from build123d import *

# Parameters (mm, degrees)
SKETCH1_R           = 22.25
BOSS_EXTRUDE1_DEPTH = 67.5
SKETCH2_R           = 8.75
BOSS_EXTRUDE2_DEPTH = 4.7
SKETCH3_R           = 2.5
BOSS_EXTRUDE3_DEPTH = 14.5
SKETCH4_R           = 2
CUT_EXTRUDE1_DEPTH  = 14.5
FILLET1_R           = 2
FILLET2_R           = 1


with BuildPart() as part:
    # Sketch1 → Boss-Extrude1 (new body)
    with BuildSketch(Plane(origin=(0, 0, 0), x_dir=(1, 0, 0), z_dir=(0, 1, 0))):
        with Locations(Location((0, 0, 0), (0, 0, 270))):
            Circle(SKETCH1_R)
    extrude(amount=BOSS_EXTRUDE1_DEPTH)

    # Sketch2 → Boss-Extrude2 (add)
    with BuildSketch(Plane(origin=(0, 67.5, 0), x_dir=(1, 0, 0), z_dir=(0, 1, 0))):
        with Locations(Location((0, 0, 0), (0, 0, 270))):
            Circle(SKETCH2_R)
    extrude(amount=BOSS_EXTRUDE2_DEPTH)

    # Sketch3 → Boss-Extrude3 (add)
    with BuildSketch(Plane(origin=(0, 72.2, 0), x_dir=(1, 0, 0), z_dir=(0, 1, 0))):
        with Locations(Location((0, 0, 0), (0, 0, 90))):
            Circle(SKETCH3_R)
    extrude(amount=BOSS_EXTRUDE3_DEPTH)

    # Sketch4 → Cut-Extrude1 (cut)
    with BuildSketch(Plane(origin=(0, 67.5, 0), x_dir=(1, 0, 0), z_dir=(0, 1, 0))):
        with Locations(Location((14.5, 0, 0), (0, 0, 270))):
            Circle(SKETCH4_R)
        with Locations(Location((-14.5, 0, 0), (0, 0, 270))):
            Circle(SKETCH4_R)
    extrude(amount=-CUT_EXTRUDE1_DEPTH, mode=Mode.SUBTRACT)

    # Fillet1
    fillet1_edges = [part.edges().sort_by_distance(p)[0] for p in [
        (0, 0, -22.25),
        (0, 67.5, -22.25),
    ]]
    fillet(fillet1_edges, radius=FILLET1_R)

    # Fillet2
    fillet2_edges = [part.edges().sort_by_distance(p)[0] for p in [
        (0, 72.2, -8.75),
    ]]
    fillet(fillet2_edges, radius=FILLET2_R)


solid = part.part
Can you work these out from the model? Positions are in its coordinate system, mm. A direction names the side the tool comes from. Coordinates: 2 decimals unless noted, no trailing zeros. Write each loop counter-clockwise with the first axis right and the second up, starting at its lowest first coordinate (ties: lowest second). Pieces come first, ordered by that corner, then holes. Notation, with made-up numbers: (76.25, 59) -> (84.25, 59) arc R27 ccw to (84.25, 98) -> close; hole circle Ø10 at (82, -32.75). An arc over 180 degrees is marked (long way). Answer as CSV lines item,"result".
1) On a 3-axis mill with a long thin cutter (end or side, diameter ignored), from which of +Z, -Z, +X, -X, +Y, -Y can I reach the whole of each face in a straight line? I mean faces 1 (the flat face through (0, 0, 0)), 2 (the cylindrical face through (2.44, 79.35, 0.54)). Say none if no direction works.
Check result:
face 1,"+Z, -Z, +X, -X, -Y"
face 2,"+Y"
2) Will these pins go through, and if not, where does the flat tip stop? P1, Ø4.5, axis at x = 15, z = 0, coming from the +Y side; P2, Ø8, axis at x = 17.5, y = 41.5, coming from the +Z side; P3, Ø10, axis at x = -4.5, z = -8, coming from the +Y side.
Check result:
P1,"y = 67.5"
P2,"z = 17.69"
P3,"y = 72.2"
3) If we section it at D-D on y = 14.5: Please give me the cut outline in (x, z).
Check result:
outline,"circle Ø44.5 at (0, 0)"
4) If I drill on line 1 (X direction, y = 56, z = 0); line 2 (Y direction, x = 7.5, z = -7); line 3 (Y direction, x = 6, z = -0.5), over which ranges is the centre line in solid material (lowest first)? Write a range as from..to.
Check result:
line 1,"-22.25..-16.5, -12.5..12.5, 16.5..22.25"
line 2,"0..67.5"
line 3,"0..72.2"
5) If we section it at B-B on x = 0: Please give me the cut outline in (y, z).
Check result:
outline,"(0, -20.25) arc R2 ccw to (2, -22.25) -> (65.5, -22.25) arc R2 ccw to (67.5, -20.25) -> (67.5, -8.75) -> (71.2, -8.75) arc R1 ccw to (72.2, -7.75) -> (72.2, -2.5) -> (86.7, -2.5) -> (86.7, 2.5) -> (72.2, 2.5) -> (72.2, 7.75) arc R1 ccw to (71.2, 8.75) -> (67.5, 8.75) -> (67.5, 20.25) arc R2 ccw to (65.5, 22.25) -> (2, 22.25) arc R2 ccw to (0, 20.25) -> close"
6) If we section it at A-A on z = 0: Please give me the cut outline in (x, y).
Check result:
outline,"(-22.25, 2) arc R2 ccw to (-20.25, 0) -> (20.25, 0) arc R2 ccw to (22.25, 2) -> (22.25, 65.5) arc R2 ccw to (20.25, 67.5) -> (16.5, 67.5) -> (16.5, 53) -> (12.5, 53) -> (12.5, 67.5) -> (8.75, 67.5) -> (8.75, 71.2) arc R1 ccw to (7.75, 72.2) -> (2.5, 72.2) -> (2.5, 86.7) -> (-2.5, 86.7) -> (-2.5, 72.2) -> (-7.75, 72.2) arc R1 ccw to (-8.75, 71.2) -> (-8.75, 67.5) -> (-12.5, 67.5) -> (-12.5, 53) -> (-16.5, 53) -> (-16.5, 67.5) -> (-20.25, 67.5) arc R2 ccw to (-22.25, 65.5) -> close"
7) If we section it at C-C on y = 79: Please give me the cut outline in (x, z).
Check result:
outline,"circle Ø5 at (0, 0)"
